Could you check a few things on this model? Use its own coordinates, in mm. A direction names the side the tool comes from. Round coordinates to 2 decimals unless told otherwise and drop trailing zeros. Write each loop counter-clockwise with the first axis right and the second up, starting at its lowest first coordinate (ties: lowest second). Pieces come first, ordered by that corner, then holes. Notation, with made-up numbers: (63.5, 81.5) -> (97.5, 81.5) arc R26 ccw to (97.5, 119.5) -> close; hole circle Ø10 at (-33.75, -6). An arc over 180 degrees is marked (long way). Return JSON: item names as keys, results as strings.
from build123d import *

# Parameters (mm, degrees)
SKETCH1_R           = 22
BOSS_EXTRUDE1_DEPTH = 36
SKETCH2_R           = 1.65
CUT_EXTRUDE1_DEPTH  = 36
CUT_EXTRUDE2_DEPTH  = 10
SKETCH4_R           = 2.3
CUT_EXTRUDE3_DEPTH  = 38
SKETCH5_R           = 5.59540043
CUT_EXTRUDE4_DEPTH  = 9


with BuildPart() as part:
    # Sketch1 → Boss-Extrude1 (new body)
    with BuildSketch(Plane(origin=(0, 0, 0), x_dir=(1, 0, 0), z_dir=(0, 1, 0))):
        Circle(SKETCH1_R)
    extrude(amount=BOSS_EXTRUDE1_DEPTH)

    # Sketch2 → Cut-Extrude1 (cut)
    with BuildSketch(Plane(origin=(0, 36, 0), x_dir=(1, 0, 0), z_dir=(0, 1, 0))):
        with Locations((-11.313708499, 11.313708499)):
            Circle(SKETCH2_R)
        with Locations((0, 16)):
            Circle(SKETCH2_R)
        with Locations((16, 0)):
            Circle(SKETCH2_R)
        with Locations((11.313708499, 11.313708499)):
            Circle(SKETCH2_R)
        with Locations((0, -16)):
            Circle(SKETCH2_R)
        with Locations((11.313708499, -11.313708499)):
            Circle(SKETCH2_R)
        with Locations((-16, 0)):
            Circle(SKETCH2_R)
        with Locations((-11.313708499, -11.313708499)):
            Circle(SKETCH2_R)
    extrude(amount=-CUT_EXTRUDE1_DEPTH, mode=Mode.SUBTRACT)

    # Sketch3 → Cut-Extrude2 (cut)
    with BuildSketch(Plane(origin=(0, 36, 0), x_dir=(1, 0, 0), z_dir=(0, 1, 0))):
        Polygon((1.321693068, -6.874091026), (6.613983991, -2.29242574), (5.292290922, 4.581665286), (-1.321693068, 6.874091026), (-6.613983991, 2.29242574), (-5.292290922, -4.581665286), align=None)
    extrude(amount=-CUT_EXTRUDE2_DEPTH, mode=Mode.SUBTRACT)

    # Sketch4 → Cut-Extrude3 (cut)
    with BuildSketch(Plane(origin=(0, 26, 0), x_dir=(1, 0, 0), z_dir=(0, 1, 0))):
        Circle(SKETCH4_R)
    extrude(amount=-CUT_EXTRUDE3_DEPTH, mode=Mode.SUBTRACT)

    # Sketch5 → Cut-Extrude4 (cut)
    with BuildSketch(Plane(origin=(0, 0, 0), x_dir=(-1, 0, 0), z_dir=(0, -1, 0))):
        Circle(SKETCH5_R)
    extrude(amount=-CUT_EXTRUDE4_DEPTH, mode=Mode.SUBTRACT)


solid = part.part
1) I want a section at D-D, the plane x = -11.5. Please give me the cut outline in (y, z) (3 decimals), and give its area (3 significant figures).
Return value:
{"outline": "(0, -18.755) -> (36, -18.755) -> (36, -12.953) -> (0, -12.953) -> close; (0, -9.674) -> (36, -9.674) -> (36, 9.674) -> (0, 9.674) -> close; (0, 12.953) -> (36, 12.953) -> (36, 18.755) -> (0, 18.755) -> close", "area": "1,110 mm²"}
2) For faces 1 (the face through (-2.032, 31.07, 5.712)), 2 (the face through (-11.671, 18.252, 12.924)), 3 (the face through (-2.4, 9, 1.2)), which set-ups out of +Z, -Z, +X, -X, +Y, -Y let a thin tool reach every point of the face, with its end or its side?
Return value:
{"face 1": "+Y", "face 2": "+Y, -Y", "face 3": "-Y"}
3) Will these pins go through, and if not, where does the flat tip stop? pin 1 Ø2 at (x, z) = (11.31, 11.31) entering from -Y; pin 2 Ø8 at (y, z) = (7, 6.5) entering from -X; pin 3 Ø5 at (y, z) = (17, -6) entering from +X; pin 4 Ø3 at (x, y) = (12, 15) entering from +Z.
Return value:
{"pin 1": "through", "pin 2": "x = -21.86", "pin 3": "x = 21.72", "pin 4": "z = 19.33"}
4) Thinking about a two-plate mould opening in Z: for faces 4 (the face through (4.44, 4.437, 3.405)), 5 (the face through (5, 0, 5)), 6 (the face through (-4.769, 17.748, 21.477)), 7 (the face through (0.89, 18.25, -17.39)), which applies, pulls with the +Z half, pulls with the -Z half, needs draft (parallel to the pull), parting line crosses it, or undercut?
Return value:
{"face 4": "undercut", "face 5": "needs draft", "face 6": "parting line crosses it", "face 7": "undercut"}
5) I want a section at C-C, the plane x = -16. Please give me the cut outline in (y, z), and give its area (3 significant figures).
Return value:
{"outline": "(0, -15.1) -> (36, -15.1) -> (36, -1.65) -> (0, -1.65) -> close; (0, 1.65) -> (36, 1.65) -> (36, 15.1) -> (0, 15.1) -> close", "area": "968 mm²"}
6) I want a section at A-A, the plane z = 16. Please give me the cut outline in (x, y), and give its area (3 significant figures).
Return value:
{"outline": "(-15.1, 0) -> (-1.65, 0) -> (-1.65, 36) -> (-15.1, 36) -> close; (1.65, 0) -> (15.1, 0) -> (15.1, 36) -> (1.65, 36) -> close", "area": "968 mm²"}
7) I want a section at B-B, the plane y = 18.5. Count the separate pieces of the cut face and the enclosed holes in it, and give its area (3 significant figures).
Return value:
{"separate pieces": "1", "enclosed holes": "9", "area": "1,440 mm²"}
8) If I drill on probe 1 along X at (y, z) = (4, 0); probe 2 along X at (y, z) = (18.25, 0); probe 3 along X at (y, z) = (17, -12), over which ranges is the centre line in solid material (lowest first)? Write a range as [from, to].
Return value:
{"probe 1": "[-22, -17.65], [-14.35, -5.6], [5.6, 14.35], [17.65, 22]", "probe 2": "[-22, -17.65], [-14.35, -2.3], [2.3, 14.35], [17.65, 22]", "probe 3": "[-18.44, -12.81], [-9.81, 9.81], [12.81, 18.44]"}
